Source: CAD feature listing. Evaluate the final solid. Frame: model axes, mm. Face numbers are marked on the shaded views. A direction names the side the tool comes from. Give positions to 0.01 mm unless a question says otherwise; leave off trailing zeros. Order: outer loops, then holes, each group sorted by start corner. A loop starts at its lowest first (then second) coordinate and runs counter-clockwise, first axis right, second up.
1) Section C-C, the plane x = 18.5. Return loops of the section in (y, z) (1 decimal).
2) Section A-A, the plane y = 0. Return loops of the section in (x, z).
3) First-contact query: P1, Ø4, axis at x = 17.5, y = 7.5, coming from the -Z side; P2, Ø2, axis at y = -6.5, z = -1, coming from the -X side; P3, Ø0.6, axis at x = 20.5, y = 9.5, coming from the +Z side; P4, Ø6, axis at x = 7, y = -4.5, coming from the +Z side. Flat tips, straight axial feed; report the tip coordinate or a pass-through.
4) Access query for the marked faces 1 and 2. Directions: +Z, -Z, +X, -X, +Y, -Y. A direction counts if a zero-diameter tool reaches every point of the face in a straight line with its end or side. Return the directions, or none.
5) Material intervals for line 1 (Z direction, x = 37.5, y = 0); line 2 (Z direction, x = 35.5, y = -5); line 3 (Y direction, x = 16.5, z = -5.5), sorted ascending.
6) Section B-B, the plane z = 0. Return loops of the section in (x, y).
```python
from build123d import *

# Parameters (mm, degrees)
F0_W     = 50.8
F0_H     = 3.175
F2_W     = 4.064
F2_H     = 2.54
F3_DEPTH = 50.801
F4_W     = 2.286
F4_H     = 4.7752
F5_DEPTH = 50.801


with BuildPart() as f1:
    # F0 (on Front) → F1 (revolve)
    with BuildSketch(Plane.XZ):
        with Locations((25.4, 9.525)):
            Rectangle(F0_W, F0_H)
    revolve(axis=Axis((25.403365, 0, 0), (1, 0, 0)))

    # F2 (on face) → F3 (cut, through all)
    with BuildSketch(Plane.YZ.offset(50.8)):
        with Locations((0, 8.6995)):
            Rectangle(F2_W, F2_H)
    extrude(amount=-F3_DEPTH, mode=Mode.SUBTRACT)

    # F4 (on face) → F5 (cut, through all)
    with BuildSketch(Plane.YZ.offset(50.8)):
        with Locations((9.9695, 0)):
            Rectangle(F4_W, F4_H)
    extrude(amount=-F5_DEPTH, mode=Mode.SUBTRACT)


solid = f1.part
```
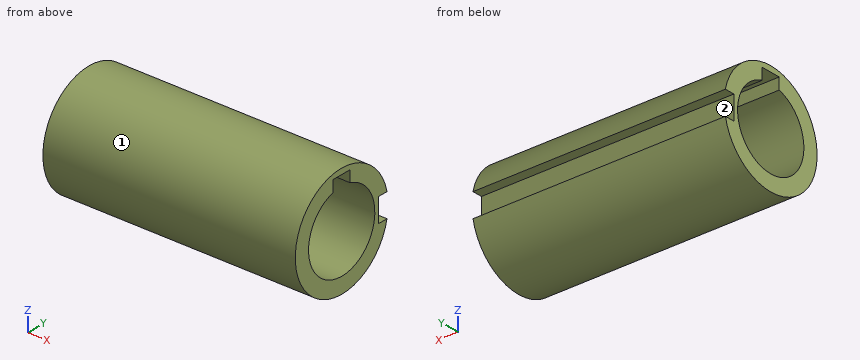
From the geometry:
1. outline: (8.8, -2.4) - (8.8, 2.4) - (10.9, 2.4) arc R11.1 ccw (long way) to (10.9, -2.4) - close; hole (-2, 7.7) arc R7.9 ccw (long way) to (2, 7.7) - (2, 10) - (-2, 10) - close
2. outline: (0, -11.11) - (50.8, -11.11) - (50.8, -7.94) - (0, -7.94) - close; (0, 9.97) - (50.8, 9.97) - (50.8, 11.11) - (0, 11.11) - close
3. P1: stops at z = -9.66
3. P2: passes through
3. P3: stops at z = 6.23
3. P4: stops at z = 11.01
4. face 1: +X, -X
4. face 2: +X, -X, +Y
5. line 1: z = -11.11 to -7.94, 9.97 to 11.11
5. line 2: z = -9.92 to -6.16, 6.16 to 9.92
5. line 3: y = -9.66 to -5.72, 5.72 to 9.66
6. outline: (0, -11.11) - (50.8, -11.11) - (50.8, -7.94) - (0, -7.94) - close; (0, 7.94) - (50.8, 7.94) - (50.8, 8.83) - (0, 8.83) - close
